```python
from build123d import *

# Parameters (mm, degrees)
BOSS_EXTRUDE1_DEPTH           = 11.5
BOSS_EXTRUDE2_START           = 11.5
SKETCH1_3_R                   = 1.5
BOSS_EXTRUDE2_DEPTH           = 2
BOSS_EXTRUDE2_DRAFT           = 1
BOSS_EXTRUDE2_PROFILE_2_DEPTH = 2
BOSS_EXTRUDE2_PROFILE_2_DRAFT = 1


with BuildPart() as part:
    # Sketch1 → Boss-Extrude1 (new body)
    with BuildSketch(Plane(origin=(0, 0, 0), x_dir=(0, 1, 0), z_dir=(0, 0, 1))):
        with BuildLine():
            Line((2, 0), (18, 0))
            ThreePointArc((18, 0), (19.414213562, 0.585786438), (20, 2))
            Line((20, 2), (20, 4))
            ThreePointArc((20, 4), (19.414213562, 5.414213562), (18, 6))
            Line((18, 6), (2, 6))
            ThreePointArc((2, 6), (0.585786438, 5.414213562), (0, 4))
            Line((0, 4), (0, 2))
            ThreePointArc((0, 2), (0.585786438, 0.585786438), (2, 0))
        make_face()
    extrude(amount=BOSS_EXTRUDE1_DEPTH)


with BuildPart() as boss_extrude2_tool:
    # Sketch1<3> → Boss-Extrude2 (with draft: the straight prism first)
    with BuildSketch(Plane(origin=(0, 0, 0), x_dir=(0, 1, 0), z_dir=(0, 0, 1)).offset(BOSS_EXTRUDE2_START)):
        with Locations((2.5, 3)):
            Circle(SKETCH1_3_R)
    extrude(amount=BOSS_EXTRUDE2_DEPTH)
    # Boss-Extrude2: the draft: its side faces are tilted about the plane it starts from
    boss_extrude2_sides = [boss_extrude2_tool.faces().sort_by_distance(p)[0] for p in [
        (-3, 1, 12.5),
    ]]
    draft(boss_extrude2_sides, Plane(origin=(0, 0, 0), x_dir=(0, 1, 0), z_dir=(0, 0, 1)).offset(BOSS_EXTRUDE2_START), BOSS_EXTRUDE2_DRAFT)


with BuildPart() as part_1:
    add(part.part)

    # Boss-Extrude2: add boss_extrude2_tool
    add(boss_extrude2_tool.part)


with BuildPart() as boss_extrude2_profile_2_tool:
    # Sketch1<3> → Boss-Extrude2 profile 2 (with draft: the straight prism first)
    with BuildSketch(Plane(origin=(0, 0, 0), x_dir=(0, 1, 0), z_dir=(0, 0, 1)).offset(BOSS_EXTRUDE2_START)):
        with Locations((17.5, 3)):
            Circle(SKETCH1_3_R)
    extrude(amount=BOSS_EXTRUDE2_PROFILE_2_DEPTH)
    # Boss-Extrude2 profile 2: the draft: its side faces are tilted about the plane it starts from
    boss_extrude2_profile_2_sides = [boss_extrude2_profile_2_tool.faces().sort_by_distance(p)[0] for p in [
        (-3, 16, 12.5),
    ]]
    draft(boss_extrude2_profile_2_sides, Plane(origin=(0, 0, 0), x_dir=(0, 1, 0), z_dir=(0, 0, 1)).offset(BOSS_EXTRUDE2_START), BOSS_EXTRUDE2_PROFILE_2_DRAFT)


with BuildPart() as part_2:
    add(part_1.part)

    # Boss-Extrude2 profile 2: add boss_extrude2_profile_2_tool
    add(boss_extrude2_profile_2_tool.part)


solid = part_2.part
```
Design review of the part built by this model. Coordinates are the model's own, in mm. A direction names the side the tool comes from. Give positions to 0.01 mm unless a question says otherwise; leave off trailing zeros. Write each loop counter-clockwise with the first axis right and the second up, starting at its lowest first coordinate (ties: lowest second). Pieces come first, ordered by that corner, then holes.
(1) Tool access review of faces 1 (the face through (-2.43, 3.87, 12.49)), 2 (the face through (-3, 2, 13.5)): name each direction out of +Z, -Z, +X, -X, +Y, -Y from which nothing blocks a thin tool from reaching the whole face with its end or side.
Checked values:
face 1: +Z
face 2: +Z, +X, -X, +Y, -Y
(2) Clearance check with a flat-ended pin moving along its axis: pin 1 Ø1 at (x, y) = (-3, 15) entering from +Z. State where the tip first meets the part, or that it passes through.
Checked values:
pin 1: stops at z = 11.5
(3) Mouldability with a two-part tool opening along Y and no side actions: class faces 3 (the face through (-3, 10, 11.5)), 4 (the face through (-5.43, 0.6, 5.67)), 5 (the face through (-3, 20, 6)), 6 (the face through (-3, 17, 13.5)) as +Y half, -Y half, draft (parallel to the pull), parting line (faces both ways), or undercut.
Checked values:
face 3: undercut
face 4: -Y half
face 5: +Y half
face 6: draft
(4) Add section A-A (z = 4). Give the boundary of the cut face in (x, y).
Checked values:
outline: (-6, 2) arc R2 ccw to (-4, 0) - (-2, 0) arc R2 ccw to (0, 2) - (0, 18) arc R2 ccw to (-2, 20) - (-4, 20) arc R2 ccw to (-6, 18) - close
(5) Wall thickness on line 1 along Z through (x, y) = (-1.7, 3.5); line 2 along Y through (x, z) = (-4.15, 5.25); line 3 along Y through (x, z) = (-4.85, 6.5): over which ranges is each line inside the solid? List them lowest first.
Checked values:
line 1: z = 0 to 11.5
line 2: y = 0.01 to 19.99
line 3: y = 0.19 to 19.81
(6) Add section C-C (x = -0.85). Give the boundary of the cut face in (y, z).
Checked values:
outline: (0.36, 0) - (19.64, 0) - (19.64, 11.5) - (0.36, 11.5) - close
(7) Add section B-B (y = 9.5). Give the boundary of the cut face in (x, z), and give its area (3 significant figures).
Checked values:
outline: (-6, 0) - (0, 0) - (0, 11.5) - (-6, 11.5) - close
area: 69.0 mm2
